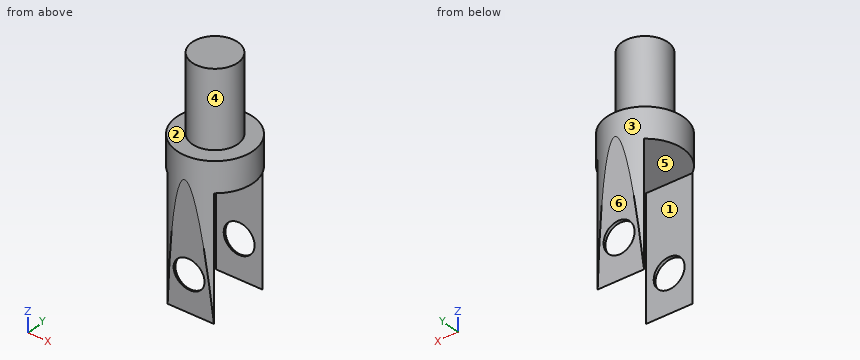
from build123d import *

# Parameters (mm, degrees)
SKETCH1_R           = 5
BOSS_EXTRUDE1_DEPTH = 20
SKETCH2_R           = 3
BOSS_EXTRUDE2_DEPTH = 10
CUT_EXTRUDE1_DEPTH  = 5
SKETCH4_W           = 16.051327138
SKETCH4_H           = 8
CUT_EXTRUDE2_DEPTH  = 5
SKETCH5_R           = 2
CUT_EXTRUDE3_DEPTH  = 5


with BuildPart() as part:
    # Sketch1 → Boss-Extrude1 (new body)
    with BuildSketch(Plane.XY):
        Circle(SKETCH1_R)
    extrude(amount=BOSS_EXTRUDE1_DEPTH)

    # Sketch2 → Boss-Extrude2 (add)
    with BuildSketch(Plane.XY.offset(20)):
        Circle(SKETCH2_R)
    extrude(amount=BOSS_EXTRUDE2_DEPTH)

    # Sketch3 → Cut-Extrude1 (cut, symmetric)
    with BuildSketch(Plane(origin=(0, 0, 0), x_dir=(0, 0, -1), z_dir=(1, 0, 0))):
        Polygon((0, 5), (-17, 5), (0, 4), align=None)
        Polygon((-17, -5), (0, -5), (0, -4), align=None)
    extrude(amount=CUT_EXTRUDE1_DEPTH, both=True, mode=Mode.SUBTRACT)

    # Sketch4 → Cut-Extrude2 (cut, symmetric)
    with BuildSketch(Plane(origin=(0, 0, 0), x_dir=(0, 0, -1), z_dir=(1, 0, 0))):
        with Locations((-8.025663569, 0)):
            Rectangle(SKETCH4_W, SKETCH4_H)
    extrude(amount=CUT_EXTRUDE2_DEPTH, both=True, mode=Mode.SUBTRACT)

    # Sketch5 → Cut-Extrude3 (cut, symmetric)
    with BuildSketch(Plane(origin=(0, 0, 0), x_dir=(1, 0, 0), z_dir=(0, 1, 0))):
        with Locations(Location((0, -5, 0), (0, 0, 90))):
            Circle(SKETCH5_R)
    extrude(amount=CUT_EXTRUDE3_DEPTH, both=True, mode=Mode.SUBTRACT)


solid = part.part
Source: CAD feature listing. Evaluate the final solid. Frame: model axes, mm. Face numbers are marked on the shaded views. A direction names the side the tool comes from. Round coordinates to 2 decimals unless told otherwise and drop trailing zeros. Loops run counter-clockwise (first coordinate to the right, second up) from the corner with the lowest first, then second, coordinate; pieces in that order, holes last. Notation, with made-up numbers: (35.25, 58.5) - (45.25, 58.5) arc R35 ccw to (45.25, 92.5) - close; hole circle Ø8 at (-36.75, -30). An arc over 180 degrees is marked (long way). Write item = value, one per line. Start each with the question number.
Item 1: Material intervals for line 1 (Z direction, x = 1, y = -3.25); line 2 (Z direction, x = 0, y = 4.3); line 3 (Y direction, x = 1.25, z = 8), sorted ascending.
Item 2: First-contact query: pin 1 Ø2 at (x, y) = (-4, 0.5) entering from +Z; pin 2 Ø1.8 at (x, z) = (0, 7) entering from +Y; pin 3 Ø4 at (x, y) = (4, 1) entering from -Z. Flat tips, straight axial feed; report the tip coordinate or a pass-through.
Item 3: Section query D-D on z = 2.5. Output: boundary loops of the cut face in (x, y).
Item 4: Section query C-C on y = 0. Output: boundary loops of the cut face in (x, z), plus the area to 3 significant figures.
Item 5: Reachability of the marked faces 1, 2 and 3 from +Z, -Z, +X, -X, +Y, -Y: full face, straight path, thin tool, end or side. Return the list, or none.
Item 6: Mould query, pull axis Y, two halves, no side actions, for the marked faces 4, 5 and 6. Classes: released by +Y, released by -Y, zero draft, split by the parting line, or undercut.
Item 7: Section query A-A on z = 7.75. Output: boundary loops of the cut face in (x, y), plus the area to 3 significant figures.
Item 8: Section query B-B on x = 0.5. Output: boundary loops of the cut face in (y, z).
Results list:
q1.line_1 = 16.05 to 20
q1.line_2 = 7 to 20
q1.line_3 = -4.47 to -4, 4 to 4.47
q2.pin_1 = 20
q2.pin_2 = 4.46
q2.pin_3 = 16.05
q3.outline = (-3, -4) arc R5 ccw to (-2.79, -4.15) - (2.79, -4.15) arc R5 ccw to (3, -4) - close; (-3, 4) - (3, 4) arc R5 ccw to (2.79, 4.15) - (-2.79, 4.15) arc R5 ccw to start
q4.outline = (-5, 16.05) - (5, 16.05) - (5, 20) - (3, 20) - (3, 30) - (-3, 30) - (-3, 20) - (-5, 20) - close
q4.area = 99.5 mm²
q5.face_1 = -Z, +X, -X
q5.face_2 = +Z
q5.face_3 = +Z, -Z
q6.face_4 = split by the parting line
q6.face_5 = undercut
q6.face_6 = released by +Y
q7.outline = (-3, -4) arc R5 ccw to (-2.27, -4.46) - (2.27, -4.46) arc R5 ccw to (3, -4) - close; (-3, 4) - (3, 4) arc R5 ccw to (2.27, 4.46) - (-2.27, 4.46) arc R5 ccw to start
q7.area = 4.85 mm²
q8.outline = (-4.97, 16.57) - (-4.41, 6.94) - (-4, 6.94) - (-4, 16.05) - (4, 16.05) - (4, 6.94) - (4.41, 6.94) - (4.97, 16.57) - (4.97, 20) - (2.96, 20) - (2.96, 30) - (-2.96, 30) - (-2.96, 20) - (-4.97, 20) - close; (-4.18, 3.06) - (-4, 0) - (-4, 3.06) - close; (4, 0) - (4.18, 3.06) - (4, 3.06) - close
